Verification items for the finished model (mm, model axes). A direction names the side the tool comes from. Round coordinates to 2 decimals unless told otherwise and drop trailing zeros. Loops run counter-clockwise (first coordinate to the right, second up) from the corner with the lowest first, then second, coordinate; pieces in that order, holes last. Notation, with made-up numbers: (19.25, 63.25) -> (74.25, 63.25) arc R30 ccw to (74.25, 101.25) -> close; hole circle Ø2 at (-19, 66.25). An arc over 180 degrees is marked (long way). Use a Markdown table: item, result. Add a question column.
```python
from build123d import *

# Parameters (mm, degrees)
PAD_DEPTH       = 11
SKETCH004_R     = 2.25
POCKET003_DEPTH = 25
SKETCH005_R     = 1.5
POCKET004_DEPTH = 5


with BuildPart() as part:
    # Sketch → Pad (new body, symmetric)
    with BuildSketch(Plane.XZ):
        Polygon((-1.5, 40), (-1.5, 0), (13.5, 0), (13.5, 9), (20.8, 9), (20.8, 14), (13.5, 14), (13.5, 40), align=None)
    extrude(amount=PAD_DEPTH, both=True)

    # Sketch004 (on Face10 of Pad) → Pocket003 (cut)
    with BuildSketch(Plane.XZ.offset(11)):
        with Locations((3.4, 32.5)):
            Circle(SKETCH004_R)
        with Locations((3.4, 7.5)):
            Circle(SKETCH004_R)
    extrude(amount=-POCKET003_DEPTH, mode=Mode.SUBTRACT)

    # Sketch005 (on Face9 of Pocket003) → Pocket004 (cut)
    with BuildSketch(Plane(origin=(0, 0, 9), x_dir=(1, 0, 0), z_dir=(0, 0, -1))):
        with Locations((16.95, 5)):
            Circle(SKETCH005_R)
        with Locations((16.95, -5)):
            Circle(SKETCH005_R)
    extrude(amount=-POCKET004_DEPTH, mode=Mode.SUBTRACT)


solid = part.part
```
1) Sectioned sample at C-C on x = 3.4. Enter the section's corners in (y, z), then the cut area to 3 significant figures.
2) Thickness scan on line 1 (Y direction, x = 16.95, z = 12.6); line 2 (Z direction, x = 3.4, y = -4.75); line 3 (X direction, y = -5, z = 12.3). Record the ranges inside material, lowest first.
3) Sectioned sample at D-D on y = 1.5. Enter the section's corners in (x, z), then the cut area to 3 significant figures.
4) Release check for a two-part mould opening along Z. For faces 4 (the face through (6, 0, 0)), 5 (the face through (20.8, 0, 11)), 6 (the face through (17, 0, 14)), 7 (the face through (4.61, -0.154, 9.397)) record: released by +Z, released by -Z, zero draft, split by the parting line, or undercut.
5) Sectioned sample at A-A on y = 5. Enter the section's corners in (x, z), then the cut area to 3 significant figures.
6) Go/stop test with flat-tipped pins: pin 1 (11 mm diameter, centred on y = -3, z = 23.5, fed in from +X); pin 2 (5 mm diameter, centred on x = 16.95, y = -5, fed in from -Z); pin 3 (3.5 mm diameter, centred on x = 16.5, y = -3.5, fed in from +Z). Record where each tip stops, or that it passes through.
7) Sectioned sample at B-B on z = 11.5. Enter the section's corners in (x, y).
8) Access from +Z, -Z, +X, -X, +Y, -Y to the whole of each face (thin tool, end or side, straight path). Record for faces 1 (the face through (17, 0, 9)), 2 (the face through (13.5, 0, 27)), 3 (the face through (18.38, -5.45, 11.46)).
Geometry results:
| question | item | result |
|---|---|---|
| 1 | outline | (-11, 0) -> (11, 0) -> (11, 5.25) -> (-11, 5.25) -> close; (-11, 9.75) -> (11, 9.75) -> (11, 30.25) -> (-11, 30.25) -> close; (-11, 34.75) -> (11, 34.75) -> (11, 40) -> (-11, 40) -> close |
| 1 | area | 682 mm^2 |
| 2 | line 1 | -11 to -6.5, -3.5 to 3.5, 6.5 to 11 |
| 2 | line 2 | 0 to 5.25, 9.75 to 30.25, 34.75 to 40 |
| 2 | line 3 | -1.5 to 15.45, 18.45 to 20.8 |
| 3 | outline | (-1.5, 0) -> (13.5, 0) -> (13.5, 9) -> (20.8, 9) -> (20.8, 14) -> (13.5, 14) -> (13.5, 40) -> (-1.5, 40) -> close; hole circle Ø4.5 at (3.4, 7.5); hole circle Ø4.5 at (3.4, 32.5) |
| 3 | area | 605 mm^2 |
| 4 | face 4 | released by -Z |
| 4 | face 5 | zero draft |
| 4 | face 6 | released by +Z |
| 4 | face 7 | undercut |
| 5 | outline | (-1.5, 0) -> (13.5, 0) -> (13.5, 9) -> (15.45, 9) -> (15.45, 14) -> (13.5, 14) -> (13.5, 40) -> (-1.5, 40) -> close; (18.45, 9) -> (20.8, 9) -> (20.8, 14) -> (18.45, 14) -> close; hole circle Ø4.5 at (3.4, 7.5); hole circle Ø4.5 at (3.4, 32.5) |
| 5 | area | 590 mm^2 |
| 6 | pin 1 | x = 13.5 |
| 6 | pin 2 | z = 9 |
| 6 | pin 3 | z = 14 |
| 7 | outline | (-1.5, -11) -> (20.8, -11) -> (20.8, 11) -> (-1.5, 11) -> close; hole circle Ø3 at (16.95, -5); hole circle Ø3 at (16.95, 5) |
| 8 | face 1 | -Z, +X, +Y, -Y |
| 8 | face 2 | +Z, +X, +Y, -Y |
| 8 | face 3 | +Z, -Z |
